Input: part model. Units: mm. Frame: model coordinates. A direction names the side the tool comes from. Coordinates: 2 decimals unless noted, no trailing zeros. Loops run counter-clockwise (first coordinate to the right, second up) from the corner with the lowest first, then second, coordinate; pieces in that order, holes last. Notation, with made-up numbers: (50.5, 37) - (84.5, 37) arc R33 cw to (84.5, 75) - close; hole circle Ø4 at (89, -1). An arc over 180 degrees is marked (long way). Use one line per item in the form item = value.
Autodesk Inventor part; units mm, degrees
ref_plane "YZ Plane" through (0, 0, 0) normal (1, 0, 0) x (0, 1, 0)
ref_plane "XZ Plane" through (0, 0, 0) normal (0, 1, 0) x (-1, 0, 0)
ref_plane "XY Plane" through (0, 0, 0) normal (0, 0, 1) x (1, 0, 0)
sketch "Sketch1" plane through (0, 0, 0) normal (0, 0, 1) x (1, 0, 0)
  line L0 (-38.1, 38.1) -> (38.1, 38.1)
  line L1 (38.1, 38.1) -> (38.1, -38.1)
  line L2 (38.1, -38.1) -> (-38.1, -38.1)
  line L3 (-38.1, -38.1) -> (-38.1, 38.1)
  circle A0 centre (0, 0) radius 20.5105
  point P0 (-31.75, 31.75)
  point P1 (31.75, 31.75)
  point P2 (31.75, -31.75)
  point P3 (-31.75, -31.75)
  dimension "d0" = 76.2
  dimension "d1" = 76.2
  dimension "d2" = 38.1
  dimension "d3" = 38.1
  dimension "d4" = 41.021
  dimension "d5" = 6.35
  dimension "d6" = 6.35
  dimension "d7" = 6.35
  dimension "d8" = 6.35
extrude "Extrusion1" add sketch "Sketch1" against normal blind 3.175
hole "Hole1" at (-31.75, 31.75, 0) at (31.75, 31.75, 0) at (31.75, -31.75, 0) at (-31.75, -31.75, 0) direction (0, 0, -1) diameter 5.08 end through all
sketch "Sketch3" plane through (0, 0, -3.175) normal (0, 0, -1) x (-1, 0, 0)
  line L0 (38.1, 38.1) -> (38.1, -38.1)
  line L1 (-38.1, -38.1) -> (-38.1, 38.1)
  line L2 (38.1, -38.1) -> (-38.1, -38.1)
  line L3 (-38.1, 38.1) -> (38.1, 38.1)
  line L4 (38.1, 38.1) -> (38.1, 34.925)
  line L5 (38.1, 34.925) -> (-38.1, 34.925)
  line L6 (-38.1, 34.925) -> (-38.1, 38.1)
  line L7 (-38.1, -34.925) -> (38.1, -34.925)
  line L8 (38.1, -34.925) -> (38.1, -38.1)
  line L9 (38.1, -38.1) -> (-38.1, -38.1)
  line L10 (-38.1, -38.1) -> (-38.1, -34.925)
  dimension "d32" = 3.175
  dimension "d33" = 3.175
extrude "Extrusion2" add sketch "Sketch3" along normal blind 21.59 contours L0 L5 L1 L3 | L0 L2 L1 L7
sketch "Sketch4" plane through (-38.1, 38.1, 0) normal (0, 1, 0) x (1, 0, 0)
  line L0 (0, 0) -> (0, 24.765)
  line L1 (0, 0) -> (76.2, 0)
  line L2 (76.2, 0) -> (76.2, 24.765)
  line L3 (6.35, 15.875) -> (31.75, 15.875)
  line L4 (31.75, 15.875) -> (31.75, 9.525)
  line L5 (31.75, 9.525) -> (6.35, 9.525)
  line L6 (6.35, 9.525) -> (6.35, 15.875)
  line L7 (44.45, 15.875) -> (69.85, 15.875)
  line L8 (69.85, 15.875) -> (69.85, 9.525)
  line L9 (69.85, 9.525) -> (44.45, 9.525)
  line L10 (44.45, 9.525) -> (44.45, 15.875)
  point P0 (38.1, 0)
  dimension "d36" = 6.35
  dimension "d37" = 9.525
  dimension "d38" = 6.35
  dimension "d39" = 6.35
  dimension "d40" = 25.4
  dimension "d41" = 6.35
  dimension "d42" = 25.4
extrude "Extrusion3" cut sketch "Sketch4" against normal through all
fillet "Fillet1" radius 3.175 16 edges at (6.35, 36.5125, -9.525) (6.35, 36.5125, -15.875) (31.75, 36.5125, -15.875) (31.75, 36.5125, -9.525) (-6.35, 36.5125, -9.525) (-6.35, 36.5125, -15.875) (-31.75, 36.5125, -15.875) (-31.75, 36.5125, -9.525) (6.35, -36.5125, -9.525) (6.35, -36.5125, -15.875) (31.75, -36.5125, -15.875) (31.75, -36.5125, -9.525) (-6.35, -36.5125, -9.525) (-6.35, -36.5125, -15.875) (-31.75, -36.5125, -15.875) (-31.75, -36.5125, -9.525)
equation "\"d38\" = d36"
equation "\"d41\" = d39"
equation "\"d42\" = d40"
properties part number "Btm Plate BD Motor mount"
Q1. Ray query, line 1 along X through (y, z) = (31.75, -1.2); line 2 along Y through (x, z) = (-11, -17.25) (3 decimals); line 3 along Y through (x, z) = (0, -1.75). Return the intervals inside material, ascending. Write a range as [from, to].
Check values:
line_1 = [-38.1, -34.29], [-29.21, 29.21], [34.29, 38.1]
line_2 = [-38.1, -34.925], [34.925, 38.1]
line_3 = [-38.1, -20.51], [20.51, 38.1]
Q2. Cut plane B-B, the plane y = 31.75. Return loops of the section in (x, z) (3 decimals), then the cut area to 3 significant figures.
Check values:
outline = (-38.1, -3.175) - (-34.29, -3.175) - (-34.29, 0) - (-38.1, 0) - close; (-29.21, -3.175) - (29.21, -3.175) - (29.21, 0) - (-29.21, 0) - close; (34.29, -3.175) - (38.1, -3.175) - (38.1, 0) - (34.29, 0) - close
area = 210 mm²
Q3. Pull-direction query (Z, two-part tool) for faces 1 (the cylindrical face through (-33.9, -33.1, -1.6)), 2 (the flat face through (19, 37, -9.525)), 3 (the flat face through (-17, 17, 0)), 4 (the flat face through (-19, -36, -15.875)); classes: pulls with the +Z half, pulls with the -Z half, needs draft (parallel to the pull), parting line crosses it, or undercut.
Check values:
face_1 = needs draft
face_2 = undercut
face_3 = pulls with the +Z half
face_4 = undercut
Q4. Set-up query: faces 5 (the cylindrical face through (-30.795, 36.49, -10.43)), 6 (the flat face through (1, 37, -24.765)). Return all of +Z, -Z, +X, -X, +Y, -Y with unobstructed straight access to the full face (end or side cutting, diameter ignored); none if empty.
Check values:
face_5 = +Y, -Y
face_6 = -Z, +X, -X, +Y, -Y
Q5. Cut plane C-C, the plane z = -21.5. Return loops of the section in (x, y) (3 decimals), then the cut area to 3 significant figures.
Check values:
outline = (-38.1, -38.1) - (38.1, -38.1) - (38.1, -34.925) - (-38.1, -34.925) - close; (-38.1, 34.925) - (38.1, 34.925) - (38.1, 38.1) - (-38.1, 38.1) - close
area = 484 mm²
Q6. Cut plane D-D, the plane x = 26.5. Return loops of the section in (y, z) (3 decimals).
Check values:
outline = (-38.1, -24.765) - (-34.925, -24.765) - (-34.925, -15.875) - (-38.1, -15.875) - close; (-38.1, -9.525) - (-34.925, -9.525) - (-34.925, -3.175) - (34.925, -3.175) - (34.925, -9.525) - (38.1, -9.525) - (38.1, 0) - (-38.1, 0) - close; (34.925, -24.765) - (38.1, -24.765) - (38.1, -15.875) - (34.925, -15.875) - close
Q7. First-contact query: P1, Ø8, axis at x = -30, y = -25.5, coming from the -Z side (3 decimals). Flat tip, straight axial feed; report the tip coordinate or a pass-through.
Check values:
P1 = -3.175
Q8. Cut plane A-A, the plane x = 0. Return loops of the section in (y, z) (1 decimal), then the cut area to 3 significant figures.
Check values:
outline = (-38.1, -24.8) - (-34.9, -24.8) - (-34.9, -3.2) - (-20.5, -3.2) - (-20.5, 0) - (-38.1, 0) - close; (20.5, -3.2) - (34.9, -3.2) - (34.9, -24.8) - (38.1, -24.8) - (38.1, 0) - (20.5, 0) - close
area = 249 mm²
